Can you work these out from the model? Positions are in its coordinate system, mm. Give positions to 0.01 mm unless a question says otherwise; leave off trailing zeros.
1. I'm going to push flat-ended pins straight in: pin 1 (2 mm diameter, centred on y = 1, z = -33.5, fed in from -X); pin 2 (2 mm diameter, centred on y = 2, z = -47, fed in from -X); pin 3 (1.1 mm diameter, centred on y = 0, z = 15, fed in from +X); pin 4 (1 mm diameter, centred on x = 4.5, y = -8.5, fed in from +Z). Where does each tip first touch, or does it pass through?
2. If I drill on probe 1 along Y at (x, z) = (0, 69.5); probe 2 along Y at (x, z) = (-6.5, -109.5); probe 3 along Y at (x, z) = (-7.25, 36.5), over which ranges is the centre line in solid material (lowest first)?
3. Thinking about a two-plate mould opening in X: for faces 1 (the flat face through (0, 3, -125)), 2 (the cylindrical face through (2.483, 0.782, -1.75)), which applies, pulls with the +X half, pulls with the -X half, needs draft (parallel to the pull), parting line crosses it, or undercut?
```python
from build123d import *

# Parameters (mm, degrees)
SKETCH3_R      = 2.6035
EXTRUDE1_DEPTH = 125


with BuildPart() as part:
    # Sketch3 → Extrude1 (new body, symmetric)
    with BuildSketch(Plane.XY):
        with BuildLine():
            Line((-1.115277175, 4.5085), (1.115277175, 4.5085))
            ThreePointArc((1.115277175, 4.5085), (2.806584872, 4.844922018), (4.240406305, 5.80297087))
            Line((4.240406305, 5.80297087), (7.148423664, 8.710988229))
            ThreePointArc((7.148423664, 8.710988229), (7.349906316, 9.772227925), (6.436353897, 10.348636575))
            Line((6.436353897, 10.348636575), (4.381960454, 10.276895575))
            ThreePointArc((4.381960454, 10.276895575), (3.239173075, 11.342562046), (4.304839546, 12.485349424))
            Line((4.304839546, 12.485349424), (5.728246175, 12.535055879))
            ThreePointArc((5.728246175, 12.535055879), (6.054756855, 12.230579745), (6.35923299, 12.557090424))
            Line((6.35923299, 12.557090424), (9.782092278, 12.676619304))
            ThreePointArc((9.782092278, 12.676619304), (10.108602958, 12.37214317), (10.413079092, 12.69865385))
            ThreePointArc((10.413079092, 12.69865385), (12.052764565, 12.052764565), (12.69865385, 10.413079092))
            ThreePointArc((12.69865385, 10.413079092), (12.37214317, 10.108602958), (12.676619304, 9.782092278))
            Line((12.676619304, 9.782092278), (12.557090424, 6.35923299))
            ThreePointArc((12.557090424, 6.35923299), (12.230579745, 6.054756855), (12.535055879, 5.728246175))
            Line((12.535055879, 5.728246175), (12.485349424, 4.304839546))
            ThreePointArc((12.485349424, 4.304839546), (11.342562046, 3.239173075), (10.276895575, 4.381960454))
            Line((10.276895575, 4.381960454), (10.348636575, 6.436353897))
            ThreePointArc((10.348636575, 6.436353897), (9.772227925, 7.349906316), (8.710988229, 7.148423664))
            Line((8.710988229, 7.148423664), (5.80297087, 4.240406305))
            ThreePointArc((5.80297087, 4.240406305), (4.844922018, 2.806584872), (4.5085, 1.115277175))
            Line((4.5085, 1.115277175), (4.5085, -1.115277175))
            ThreePointArc((4.5085, -1.115277175), (4.844922018, -2.806584872), (5.80297087, -4.240406305))
            Line((5.80297087, -4.240406305), (8.710988229, -7.148423664))
            ThreePointArc((8.710988229, -7.148423664), (9.772227925, -7.349906316), (10.348636575, -6.436353897))
            Line((10.348636575, -6.436353897), (10.276895575, -4.381960454))
            ThreePointArc((10.276895575, -4.381960454), (11.342562046, -3.239173075), (12.485349424, -4.304839546))
            Line((12.485349424, -4.304839546), (12.535055879, -5.728246175))
            ThreePointArc((12.535055879, -5.728246175), (12.230579745, -6.054756855), (12.557090424, -6.35923299))
            Line((12.557090424, -6.35923299), (12.676619304, -9.782092278))
            ThreePointArc((12.676619304, -9.782092278), (12.37214317, -10.108602958), (12.69865385, -10.413079092))
            ThreePointArc((12.69865385, -10.413079092), (12.052764565, -12.052764565), (10.413079092, -12.69865385))
            ThreePointArc((10.413079092, -12.69865385), (10.108602958, -12.37214317), (9.782092278, -12.676619304))
            Line((9.782092278, -12.676619304), (6.35923299, -12.557090424))
            ThreePointArc((6.35923299, -12.557090424), (6.054756855, -12.230579745), (5.728246175, -12.535055879))
            Line((5.728246175, -12.535055879), (4.304839546, -12.485349424))
            ThreePointArc((4.304839546, -12.485349424), (3.239173075, -11.342562046), (4.381960454, -10.276895575))
            Line((4.381960454, -10.276895575), (6.436353897, -10.348636575))
            ThreePointArc((6.436353897, -10.348636575), (7.349906316, -9.772227925), (7.148423664, -8.710988229))
            Line((7.148423664, -8.710988229), (4.240406305, -5.80297087))
            ThreePointArc((4.240406305, -5.80297087), (2.806584872, -4.844922018), (1.115277175, -4.5085))
            Line((1.115277175, -4.5085), (-1.115277175, -4.5085))
            ThreePointArc((-1.115277175, -4.5085), (-2.806584872, -4.844922018), (-4.240406305, -5.80297087))
            Line((-4.240406305, -5.80297087), (-7.148423664, -8.710988229))
            ThreePointArc((-7.148423664, -8.710988229), (-7.349906316, -9.772227925), (-6.436353897, -10.348636575))
            Line((-6.436353897, -10.348636575), (-4.381960454, -10.276895575))
            ThreePointArc((-4.381960454, -10.276895575), (-3.239173075, -11.342562046), (-4.304839546, -12.485349424))
            Line((-4.304839546, -12.485349424), (-5.728246175, -12.535055879))
            ThreePointArc((-5.728246175, -12.535055879), (-6.054756855, -12.230579745), (-6.35923299, -12.557090424))
            Line((-6.35923299, -12.557090424), (-9.782092278, -12.676619304))
            ThreePointArc((-9.782092278, -12.676619304), (-10.108602958, -12.37214317), (-10.413079092, -12.69865385))
            ThreePointArc((-10.413079092, -12.69865385), (-12.052764565, -12.052764565), (-12.69865385, -10.413079092))
            ThreePointArc((-12.69865385, -10.413079092), (-12.37214317, -10.108602958), (-12.676619304, -9.782092278))
            Line((-12.676619304, -9.782092278), (-12.557090424, -6.35923299))
            ThreePointArc((-12.557090424, -6.35923299), (-12.230579745, -6.054756855), (-12.535055879, -5.728246175))
            Line((-12.535055879, -5.728246175), (-12.485349424, -4.304839546))
            ThreePointArc((-12.485349424, -4.304839546), (-11.342562046, -3.239173075), (-10.276895575, -4.381960454))
            Line((-10.276895575, -4.381960454), (-10.348636575, -6.436353897))
            ThreePointArc((-10.348636575, -6.436353897), (-9.772227925, -7.349906316), (-8.710988229, -7.148423664))
            Line((-8.710988229, -7.148423664), (-5.80297087, -4.240406305))
            ThreePointArc((-5.80297087, -4.240406305), (-4.844922018, -2.806584872), (-4.5085, -1.115277175))
            Line((-4.5085, -1.115277175), (-4.5085, 1.115277175))
            ThreePointArc((-4.5085, 1.115277175), (-4.844922018, 2.806584872), (-5.80297087, 4.240406305))
            Line((-5.80297087, 4.240406305), (-8.710988229, 7.148423664))
            ThreePointArc((-8.710988229, 7.148423664), (-9.772227925, 7.349906316), (-10.348636575, 6.436353897))
            Line((-10.348636575, 6.436353897), (-10.276895575, 4.381960454))
            ThreePointArc((-10.276895575, 4.381960454), (-11.342562046, 3.239173075), (-12.485349424, 4.304839546))
            Line((-12.485349424, 4.304839546), (-12.535055879, 5.728246175))
            ThreePointArc((-12.535055879, 5.728246175), (-12.230579745, 6.054756855), (-12.557090424, 6.35923299))
            Line((-12.557090424, 6.35923299), (-12.676619304, 9.782092278))
            ThreePointArc((-12.676619304, 9.782092278), (-12.37214317, 10.108602958), (-12.69865385, 10.413079092))
            ThreePointArc((-12.69865385, 10.413079092), (-12.052764565, 12.052764565), (-10.413079092, 12.69865385))
            ThreePointArc((-10.413079092, 12.69865385), (-10.108602958, 12.37214317), (-9.782092278, 12.676619304))
            Line((-9.782092278, 12.676619304), (-6.35923299, 12.557090424))
            ThreePointArc((-6.35923299, 12.557090424), (-6.054756855, 12.230579745), (-5.728246175, 12.535055879))
            Line((-5.728246175, 12.535055879), (-4.304839546, 12.485349424))
            ThreePointArc((-4.304839546, 12.485349424), (-3.239173075, 11.342562046), (-4.381960454, 10.276895575))
            Line((-4.381960454, 10.276895575), (-6.436353897, 10.348636575))
            ThreePointArc((-6.436353897, 10.348636575), (-7.349906316, 9.772227925), (-7.148423664, 8.710988229))
            Line((-7.148423664, 8.710988229), (-4.240406305, 5.80297087))
            ThreePointArc((-4.240406305, 5.80297087), (-2.806584872, 4.844922018), (-1.115277175, 4.5085))
        make_face()
        Circle(SKETCH3_R, mode=Mode.SUBTRACT)
    extrude(amount=EXTRUDE1_DEPTH, both=True)


solid = part.part
```
Checks:
1. pin 1: stops at x = -4.6
1. pin 2: stops at x = -4.93
1. pin 3: stops at x = 4.51
1. pin 4: passes through
2. probe 1: y = -4.51 to -2.6, 2.6 to 4.51
2. probe 2: y = -12.56 to -10.35, -8.06 to -4.94, 4.94 to 8.06, 10.35 to 12.56
2. probe 3: y = -12.59 to -9.95, -8.83 to -5.69, 5.69 to 8.83, 9.95 to 12.59
3. face 1: needs draft
3. face 2: undercut
